The listing builds one solid part. Answer for the finished solid, in the listing's coordinates (mm). Round coordinates to 2 decimals unless told otherwise and drop trailing zeros. Order: outer loops, then holes, each group sorted by start corner. A loop starts at its lowest first (then second) coordinate and runs counter-clockwise, first axis right, second up. Notation, with made-up numbers: (-4, -33.5) -> (14, -33.5) arc R3 ccw to (14, -29.5) -> close; hole circle Ø9 at (23, 55). An arc over 180 degrees is marked (long way). Answer in a Markdown table with one row per item. Add a question column.
```python
from build123d import *

# Parameters (mm, degrees)
SKETCH1_W           = 72
SKETCH1_H           = 40
SKETCH1_R           = 2
SKETCH1_R_2         = 1.5
BOSS_EXTRUDE1_DEPTH = 3.175
FILLET1_SIZE        = 5


with BuildPart() as part:
    # Sketch1 → Boss-Extrude1 (new body)
    with BuildSketch(Plane(origin=(0, 0, 0), x_dir=(1, 0, 0), z_dir=(0, 1, 0))):
        with Locations((36, 20)):
            Rectangle(SKETCH1_W, SKETCH1_H)
        with Locations(Location((20, 24, 0), (0, 0, 270))):
            Circle(SKETCH1_R, mode=Mode.SUBTRACT)
        with Locations(Location((20, 16, 0), (0, 0, 270))):
            Circle(SKETCH1_R, mode=Mode.SUBTRACT)
        with Locations(Location((52, 24, 0), (0, 0, 270))):
            Circle(SKETCH1_R, mode=Mode.SUBTRACT)
        with Locations(Location((52, 16, 0), (0, 0, 270))):
            Circle(SKETCH1_R, mode=Mode.SUBTRACT)
        with Locations(Location((7.5, 32, 0), (0, 0, 270))):
            Circle(SKETCH1_R_2, mode=Mode.SUBTRACT)
        with Locations(Location((7.5, 8, 0), (0, 0, 270))):
            Circle(SKETCH1_R_2, mode=Mode.SUBTRACT)
        with Locations(Location((64.5, 8, 0), (0, 0, 270))):
            Circle(SKETCH1_R_2, mode=Mode.SUBTRACT)
        with Locations(Location((64.5, 32, 0), (0, 0, 270))):
            Circle(SKETCH1_R_2, mode=Mode.SUBTRACT)
    extrude(amount=BOSS_EXTRUDE1_DEPTH)

    # Fillet1
    # a fillet whose section is not a circle: 5 mm, written as the material it takes off along each edge
    with BuildSketch(Plane(origin=(0, -12.5, -40), x_dir=(1, 0, 0), z_dir=(0, 1, 0)), Plane(origin=(72, -12.5, 0), x_dir=(-1, 0, 0), z_dir=(0, 1, 0)), Plane(origin=(72, -12.5, -40), x_dir=(0, 0, 1), z_dir=(0, 1, 0))) as fillet1_piece_1:
        with BuildLine():
            add(Edge.make_bspline([(FILLET1_SIZE, 0), (FILLET1_SIZE * 0.831801948466, 0), (FILLET1_SIZE * 0.663603896932, 0), (FILLET1_SIZE * 0.292893218813, -FILLET1_SIZE * 0.0716919198361), (FILLET1_SIZE * 0.0716919198361, -FILLET1_SIZE * 0.292893218813), (0, -FILLET1_SIZE * 0.663603896932), (0, -FILLET1_SIZE * 0.831801948466), (0, -FILLET1_SIZE)], knots=[0, 0, 0, 0, 0, 0, 0.5, 0.5, 1, 1, 1, 1, 1, 1], degree=5))
            Line((0, -FILLET1_SIZE), (0, 0))
            Line((0, 0), (FILLET1_SIZE, 0))
        make_face()
    extrude(amount=28.175, mode=Mode.SUBTRACT)
    with BuildSketch(Plane(origin=(0, -12.5, 0), x_dir=(1, 0, 0), z_dir=(0, 1, 0))) as fillet1_piece_2:
        with BuildLine():
            add(Edge.make_bspline([(FILLET1_SIZE, 0), (FILLET1_SIZE * 0.831801948466, 0), (FILLET1_SIZE * 0.663603896932, 0), (FILLET1_SIZE * 0.292893218813, FILLET1_SIZE * 0.0716919198361), (FILLET1_SIZE * 0.0716919198361, FILLET1_SIZE * 0.292893218813), (0, FILLET1_SIZE * 0.663603896932), (0, FILLET1_SIZE * 0.831801948466), (0, FILLET1_SIZE)], knots=[0, 0, 0, 0, 0, 0, 0.5, 0.5, 1, 1, 1, 1, 1, 1], degree=5))
            Line((0, FILLET1_SIZE), (0, 0))
            Line((0, 0), (FILLET1_SIZE, 0))
        make_face()
    extrude(amount=28.175, mode=Mode.SUBTRACT)


solid = part.part
```
Item 1: The part is cut by section B-B, the plane x = 7.5. Give the vertices of the cut face in (y, z) (3 decimals), and give its area (3 significant figures).
Item 2: The part is cut by section C-C, the plane y = 1.2. State how many separate pieces and enclosed holes the cut face has, and give its area (3 significant figures).
Item 3: Find the intervals of material crossed by probe 1 along Z at (x, y) = (64.5, 1.7); probe 2 along Z at (x, y) = (65.5, 2.6); probe 3 along X at (y, z) = (1.3, -8), in increasing order. Write a range as [from, to].
Item 4: Flat-ended cylindrical pins translate along their axes: P1, Ø2.5, axis at x = 64.5, z = -8, coming from the -Y side; P2, Ø5, axis at x = 20, z = -16, coming from the -Y side. Find the tip coordinate at first contact, or state that the pin passes through.
Item 5: The part is cut by section A-A, the plane z = -16. Give the vertices of the cut face in (x, y) (3 decimals), and give its area (3 significant figures).
Item 6: For a pull along X with two mould halves and no side action, classify faces 1 (the face through (35, 3.175, -20)), 2 (the face through (6.6, 1.6, -33.2)), 3 (the face through (72, 2, -20)), 4 (the face through (0, 2, -20)) as released by +X, released by -X, zero draft, split by the parting line, or undercut.
Resolved:
| question | item | result |
|---|---|---|
| 1 | outline | (0, -40) -> (3.175, -40) -> (3.175, -33.5) -> (0, -33.5) -> close; (0, -30.5) -> (3.175, -30.5) -> (3.175, -9.5) -> (0, -9.5) -> close; (0, -6.5) -> (3.175, -6.5) -> (3.175, 0) -> (0, 0) -> close |
| 1 | area | 108 mm2 |
| 2 | separate pieces | 1 |
| 2 | enclosed holes | 8 |
| 2 | area | 2,790 mm2 |
| 3 | probe 1 | [-40, -33.5], [-30.5, -9.5], [-6.5, 0] |
| 3 | probe 2 | [-40, -33.12], [-30.88, -9.12], [-6.88, 0] |
| 3 | probe 3 | [0, 6], [9, 63], [66, 72] |
| 4 | P1 | through |
| 4 | P2 | y = 0 |
| 5 | outline | (0, 0) -> (18, 0) -> (18, 3.175) -> (0, 3.175) -> close; (22, 0) -> (50, 0) -> (50, 3.175) -> (22, 3.175) -> close; (54, 0) -> (72, 0) -> (72, 3.175) -> (54, 3.175) -> close |
| 5 | area | 203 mm2 |
| 6 | face 1 | zero draft |
| 6 | face 2 | undercut |
| 6 | face 3 | released by +X |
| 6 | face 4 | released by -X |
